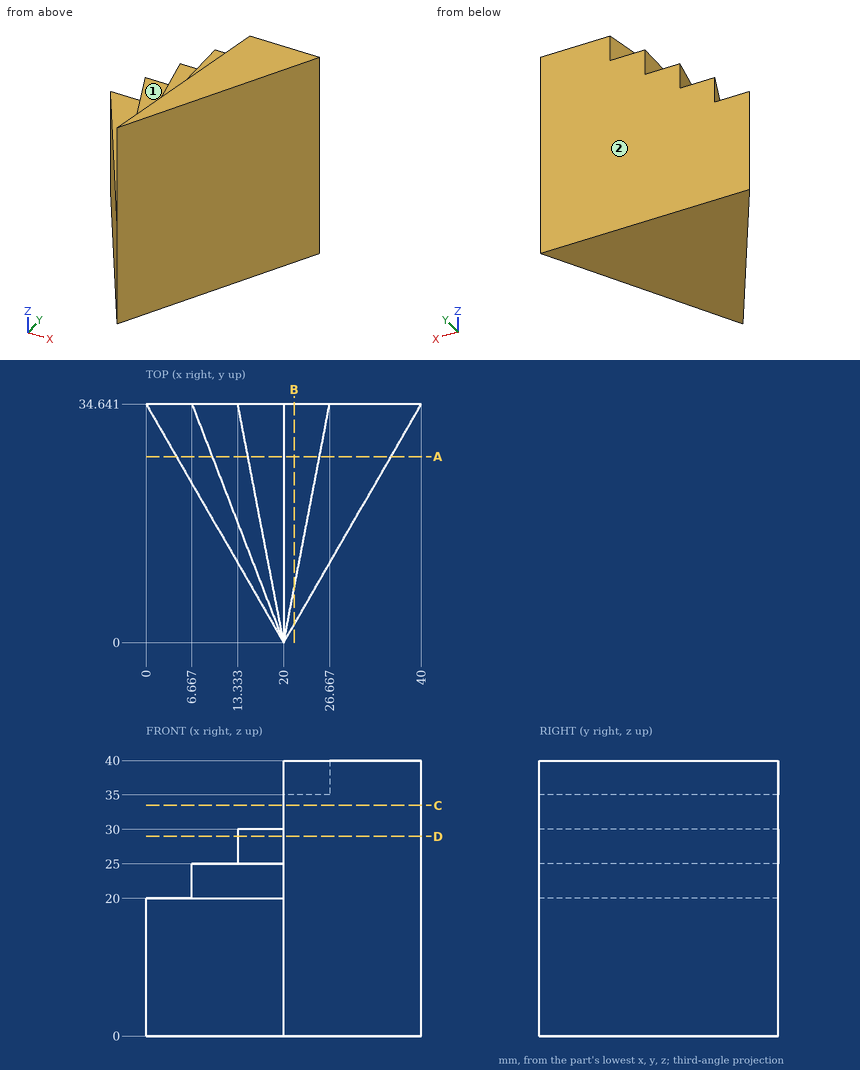
For this review, use the dimensioned drawing (mm, ordinates from the lowest corner) and the shaded views. A direction names the side the tool comes from. Give positions to 0.01 mm unless a question says otherwise; leave off trailing zeros. Write each loop counter-clockwise with the first axis right and the second up, starting at its lowest first coordinate (ties: lowest second). Pieces come first, ordered by that corner, then holes.
(1) Consider section B-B, the plane x = 21.5. Give the boundary of the cut face in (y, z).
(2) To check wall thickness, follow L1, parallel to Z at x = 11, y = 24; L2, parallel to Z at x = 11, y = 16.5; L3, parallel to Y at x = 23, z = 22 (1 decimal). State the ranges of each line that lie inside material, in increasing order.
(3) For P1, Ø10, axis at x = 13, y = 24, coming from the +Z side; P2, Ø6, axis at y = 15.5, z = 24, coming from the +X side; P3, Ø4, axis at y = 15, z = 17.5, coming from the +X side (1 decimal); P4, Ø8, axis at x = 12, z = 35, coming from the -Y side, all flat-tipped, find the tip position at first contact; note any pin that passes through.
(4) Consider section A-A, the plane y = 27. Give the boundary of the cut face in (x, z).
(5) Consider section D-D, the plane z = 29. Give the boundary of the cut face in (x, y).
(6) Tool access review of the marked faces 1 and 2: name each direction out of +Z, -Z, +X, -X, +Y, -Y from which nothing blocks a thin tool from reaching the whole face with its end or side.
(7) Consider section C-C, the plane z = 33.5. Give the boundary of the cut face in (x, y).
Returned:
1. outline: (2.6, 0) - (34.64, 0) - (34.64, 35) - (7.79, 35) - (7.79, 40) - (2.6, 40) - close
2. L1: z = 0 to 25
2. L2: z = 0 to 20
2. L3: y = 5.2 to 34.6
3. P1: stops at z = 30
3. P2: stops at x = 30.68
3. P3: stops at x = 29.8
3. P4: passes through
4. outline: (4.41, 0) - (35.59, 0) - (35.59, 40) - (25.2, 40) - (25.2, 35) - (20, 35) - (20, 30) - (14.8, 30) - (14.8, 25) - (9.61, 25) - (9.61, 20) - (4.41, 20) - close
5. outline: (13.33, 34.64) - (20, 0) - (40, 34.64) - close
6. face 1: +Z, -X, -Y
6. face 2: +Z, -Z, +X, -X, +Y
7. outline: (20, 0) - (40, 34.64) - (20, 34.64) - close
